from build123d import *

# Parameters (mm, degrees)
SKETCH1_W           = 6.35
SKETCH1_H           = 12.7
SKETCH1_R           = 0.79375
BOSS_EXTRUDE1_DEPTH = 6.35
CUT_EXTRUDE1_START  = 6.35
SKETCH1_3_R         = 0.79375
CUT_EXTRUDE1_DEPTH  = 1.27


with BuildPart() as part:
    # Sketch1 → Boss-Extrude1 (new body)
    with BuildSketch(Plane.XY):
        Rectangle(SKETCH1_W, SKETCH1_H)
        with Locations((1.058333333, 0)):
            Circle(SKETCH1_R, mode=Mode.SUBTRACT)
        with Locations((-1.058333333, 0)):
            Circle(SKETCH1_R, mode=Mode.SUBTRACT)
        with Locations((0, 2.116666667)):
            Circle(SKETCH1_R, mode=Mode.SUBTRACT)
        with Locations((-1.058333333, 0)):
            Circle(SKETCH1_R)
        with Locations((0, 2.116666667)):
            Circle(SKETCH1_R)
        with Locations((1.058333333, 0)):
            Circle(SKETCH1_R)
    extrude(amount=BOSS_EXTRUDE1_DEPTH)

    # Sketch1<3> → Cut-Extrude1 (cut)
    with BuildSketch(Plane.XY.offset(CUT_EXTRUDE1_START)):
        with Locations((-1.058333333, 0)):
            Circle(SKETCH1_3_R)
        with Locations((0, 2.116666667)):
            Circle(SKETCH1_3_R)
        with Locations((1.058333333, 0)):
            Circle(SKETCH1_3_R)
    extrude(amount=-CUT_EXTRUDE1_DEPTH, mode=Mode.SUBTRACT)


solid = part.part
The listing builds one solid part. Answer for the finished solid, in the listing's coordinates (mm). A direction names the side the tool comes from. Round coordinates to 2 decimals unless told otherwise and drop trailing zeros. Write each loop counter-clockwise with the first axis right and the second up, starting at its lowest first coordinate (ties: lowest second). Pieces come first, ordered by that corner, then holes. Notation, with made-up numbers: (70.25, 46.25) - (87.25, 46.25) arc R25 cw to (87.25, 74.25) - close; hole circle Ø2 at (66, -3.75). An arc over 180 degrees is marked (long way). Use a Markdown table: item, result. Add a question column.
1. For a pull along X with two mould halves and no side action, classify faces 3 (the face through (0, 0, 6.35)), 4 (the face through (-3.175, 0, 3)), 5 (the face through (-0.17, 1.34, 5.72)) as +X half, -X half, draft (parallel to the pull), parting line (faces both ways), or undercut.
2. Consider line 1 (Y direction, x = 0, z = 5.5); line 2 (Z direction, x = 0.25, y = 2.5). Determine where each line is inside the solid, lowest interval first.
3. The part is cut by section A-A (y = 0). Write down the section's boundary in (x, z) (3 decimals).
4. The part is cut by section B-B (x = 0). Write down the section's boundary in (y, z), and give its area (3 significant figures).
5. A flat-ended cylindrical pin translates along its axis: P1, Ø0.5, axis at x = 0, y = 2, coming from the +Z side. Find the tip coordinate at first contact, or state that the pin passes through.
6. The part is cut by section C-C (x = 1.25). Write down the section's boundary in (y, z).
7. A tool of negligible diameter and unlimited length cuts with its end or side. For faces 1 (the face through (0, 6.35, 3)), 2 (the face through (-1, 0, 5.08)), from which of +Z, -Z, +X, -X, +Y, -Y can it reach the whole face along a straight path? Write none if from no direction.
Reported:
| question | item | result |
|---|---|---|
| 1 | face 3 | draft |
| 1 | face 4 | -X half |
| 1 | face 5 | undercut |
| 2 | line 1 | -6.35 to 1.32, 2.91 to 6.35 |
| 2 | line 2 | 0 to 5.08 |
| 3 | outline | (-3.175, 0) - (3.175, 0) - (3.175, 6.35) - (1.852, 6.35) - (1.852, 5.08) - (0.265, 5.08) - (0.265, 6.35) - (-0.265, 6.35) - (-0.265, 5.08) - (-1.852, 5.08) - (-1.852, 6.35) - (-3.175, 6.35) - close |
| 4 | outline | (-6.35, 0) - (6.35, 0) - (6.35, 6.35) - (2.91, 6.35) - (2.91, 5.08) - (1.32, 5.08) - (1.32, 6.35) - (-6.35, 6.35) - close |
| 4 | area | 78.6 mm^2 |
| 5 | P1 | z = 5.08 |
| 6 | outline | (-6.35, 0) - (6.35, 0) - (6.35, 6.35) - (0.77, 6.35) - (0.77, 5.08) - (-0.77, 5.08) - (-0.77, 6.35) - (-6.35, 6.35) - close |
| 7 | face 1 | +Z, -Z, +X, -X, +Y |
| 7 | face 2 | +Z |
